Part model, mm, in its own coordinate system. A direction names the side the tool comes from. Round coordinates to 2 decimals unless told otherwise and drop trailing zeros. Order: outer loops, then holes, each group sorted by start corner. A loop starts at its lowest first (then second) coordinate and runs counter-clockwise, first axis right, second up. Notation, with made-up numbers: (20.5, 82) - (67.5, 82) arc R20 ccw to (67.5, 89) - close; hole circle Ø11 at (37.5, 73). An arc over 180 degrees is marked (long way). Return JSON: item names as keys, results as strings. Group by question number.
Item 1: Saw through at D-D on z = 8. List the corners of the cut face in (x, y).
Item 2: Drop flat-ended pins along their axis: pin 1 (10 mm diameter, centred on y = -5, z = 39, fed in from +X); pin 2 (12 mm diameter, centred on y = 0, z = 41, fed in from +X); pin 3 (12 mm diameter, centred on x = -17.5, y = -18.5, fed in from +Z); pin 4 (5.5 mm diameter, centred on x = 0.05, y = -0.3, fed in from -Z). Give the stop position or say it passes through.
Item 3: Tool access for faces 4 (the face through (-125, -8, 5)), 5 (the face through (-9.95, -18, 2)), 6 (the face through (-110.201, -7.557, 23.623)): list every direction of +Z, -Z, +X, -X, +Y, -Y with a clear straight run to the whole face (end or side of a thin tool).
Item 4: Two-plate mould, pull along X, no slides. Class faces 1 (the face through (-68, -8, 42.775)), 2 (the face through (10.05, 0, 2)), 3 (the face through (-2.3, -0.2, 0)): released by +X, released by -X, zero draft, split by the parting line, or undercut.
Item 5: Saw through at C-C on x = -4. List the corners of the cut face in (y, z), and give its area (3 significant figures).
Item 6: Probe probe 1 along Z at (x, y) = (-70, -5.5); probe 2 along X at (y, z) = (-4, 38.5); probe 3 along X at (y, z) = (-17.5, 30). List the from-to ranges inside material, lowest first.
Item 7: Saw through at B-B on y = 7. List the corners of the cut face in (x, z).
Item 8: Saw through at A-A on z = 20. List the corners of the cut face in (x, y), and give its area (3 significant figures).
```python
from build123d import *

# Parameters (mm, degrees)
ESQUISSE2_W             = 20
ESQUISSE2_H             = 20
BOSS_EXTRU_1_DEPTH      = 5
ESQUISSE3_R             = 2.2
ENL_V_MAT_EXTRU_1_DEPTH = 5
BOSS_EXTRU_2_DEPTH      = 35


with BuildPart() as part:
    # Esquisse2 → Boss.-Extru.1 (new body)
    with BuildSketch(Plane.XY):
        with Locations((0.050251256, -0.301507538)):
            Rectangle(ESQUISSE2_W, ESQUISSE2_H)
    extrude(amount=BOSS_EXTRU_1_DEPTH)

    # Esquisse3 → Enlèv. mat.-Extru.1 (cut)
    with BuildSketch(Plane.XY.offset(5)):
        with Locations((0.050251256, -0.301507538)):
            Circle(ESQUISSE3_R)
    extrude(amount=-ENL_V_MAT_EXTRU_1_DEPTH, mode=Mode.SUBTRACT)

    # Esquisse4 → Boss.-Extru.2 (add)
    with BuildSketch(Plane(origin=(0, 9.698492462, 0), x_dir=(1, 0, 0), z_dir=(0, 1, 0))):
        Polygon((-9.949748744, -5), (-35.398476961, -47.775171076), (-100.606984649, -47.775171076), (-128.128833484, -5), (-122.183304286, -5), (-97.878490958, -42.775171076), (-37.511283693, -42.775171076), (-9.949748744, 0), align=None)
    extrude(amount=-BOSS_EXTRU_2_DEPTH)


solid = part.part
```
Filled in:
{
 "1": {"outline": "(-126.2, -25.3) - (-120.25, -25.3) - (-120.25, 9.7) - (-126.2, 9.7) - close; (-15.1, -25.3) - (-11.73, -25.3) - (-11.73, 9.7) - (-15.1, 9.7) - close"},
 "2": {"pin 1": "stops at x = -27.2", "pin 2": "stops at x = -27.8", "pin 3": "stops at z = 27.78", "pin 4": "stops at z = 0"},
 "3": {"face 4": "-Z, -X, +Y, -Y", "face 5": "+Z, -Z, +X, -Y", "face 6": "-Z, +Y, -Y"},
 "4": {"face 1": "undercut", "face 2": "released by +X", "face 3": "zero draft"},
 "5": {"outline": "(-10.3, 0) - (9.7, 0) - (9.7, 5) - (-10.3, 5) - close", "area": "100 mm^2"},
 "6": {"probe 1": "z = 42.78 to 47.78", "probe 2": "x = -106.57 to -100.63, -34.76 to -29.88", "probe 3": "x = -112.04 to -106.1, -29.28 to -24.82"},
 "7": {"outline": "(-128.13, 5) - (-122.18, 5) - (-97.88, 42.78) - (-37.51, 42.78) - (-9.95, 0) - (10.05, 0) - (10.05, 5) - (-9.95, 5) - (-35.4, 47.78) - (-100.61, 47.78) - close"},
 "8": {"outline": "(-118.48, -25.3) - (-112.53, -25.3) - (-112.53, 9.7) - (-118.48, 9.7) - close; (-22.84, -25.3) - (-18.87, -25.3) - (-18.87, 9.7) - (-22.84, 9.7) - close", "area": "347 mm^2"}
}
